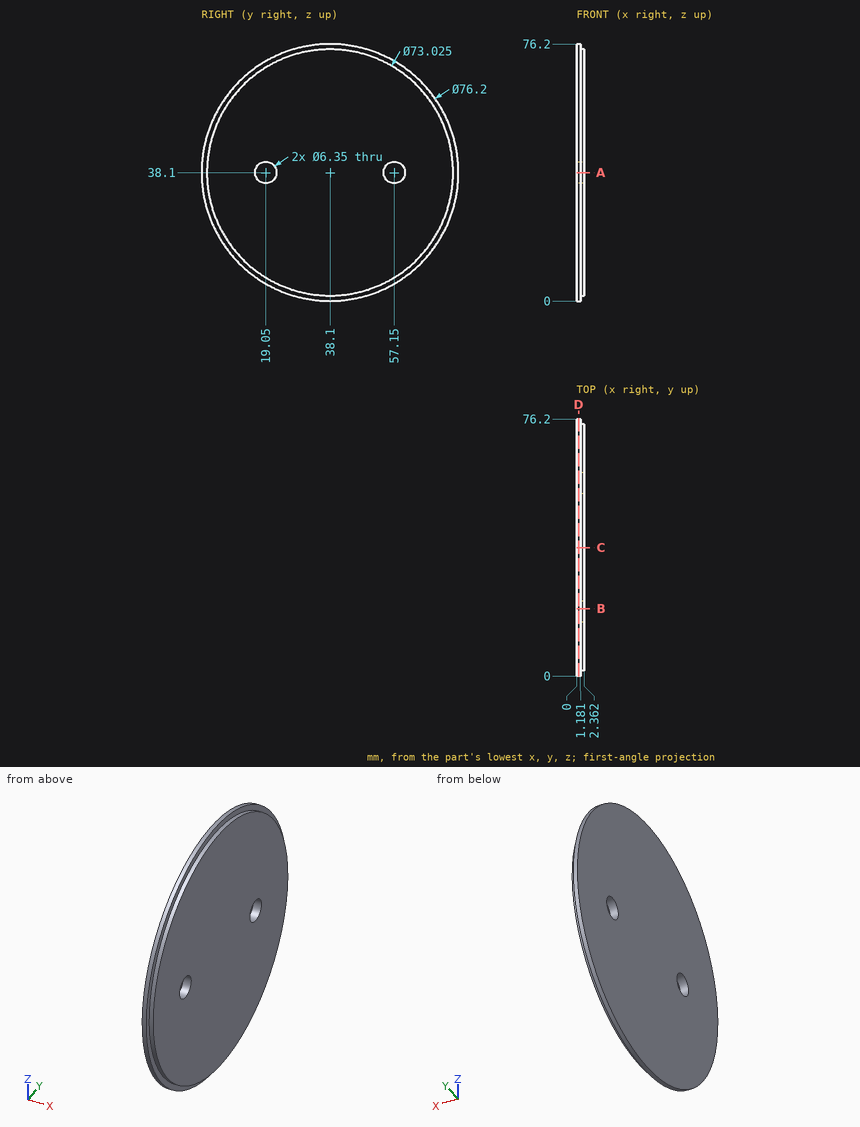
For this review, use the dimensioned drawing (mm, ordinates from the lowest corner) and the shaded views. Round coordinates to 2 decimals unless told otherwise and drop trailing zeros. Write each loop counter-clockwise with the first axis right and the second up, starting at its lowest first coordinate (ties: lowest second). Pieces come first, ordered by that corner, then holes. Notation, with made-up numbers: (84.25, 38.5) -> (121.25, 38.5) arc R35 cw to (121.25, 71.5) -> close; hole circle Ø4 at (-15.5, 87.25). An arc over 180 degrees is marked (long way). Use one line per item in the form item = value.
Q1. Consider section C-C (y = 38.1). State the section outline as (x, z) points.
Resolved:
outline = (0, 0) -> (1.18, 0) -> (1.18, 1.59) -> (2.36, 1.59) -> (2.36, 74.61) -> (1.18, 74.61) -> (1.18, 76.2) -> (0, 76.2) -> close
Q2. Consider section D-D (x = 0.6). State the section outline as (y, z) points (3 decimals), then the cut area to 3 significant figures.
Resolved:
outline = circle Ø76.2 at (38.1, 38.1); hole circle Ø6.35 at (19.05, 38.1); hole circle Ø6.35 at (57.15, 38.1)
area = 4,500 mm²
Q3. To check wall thickness, follow probe 1 along Y at (x, z) = (1.25, 38.1) (1 decimal); probe 2 along Y at (x, z) = (0.8, 38.1) (3 decimals); probe 3 along Z at (x, y) = (0.5, 18.5). State the ranges of each line that lie inside material, in increasing order. Write a range as from..to.
Resolved:
probe_1 = 1.6..15.9, 22.2..54, 60.3..74.6
probe_2 = 0..15.875, 22.225..53.975, 60.325..76.2
probe_3 = 5.43..34.97, 41.23..70.77
Q4. Consider section B-B (y = 20). State the section outline as (x, z) points, then the cut area to 3 significant figures.
Resolved:
outline = (0, 4.57) -> (1.18, 4.57) -> (1.18, 6.39) -> (2.36, 6.39) -> (2.36, 35.07) -> (0, 35.07) -> close; (0, 41.13) -> (2.36, 41.13) -> (2.36, 69.81) -> (1.18, 69.81) -> (1.18, 71.63) -> (0, 71.63) -> close
area = 140 mm²
Q5. Consider section A-A (z = 38.1). State the section outline as (x, y) points (1 decimal).
Resolved:
outline = (0, 0) -> (1.2, 0) -> (1.2, 1.6) -> (2.4, 1.6) -> (2.4, 15.9) -> (0, 15.9) -> close; (0, 22.2) -> (2.4, 22.2) -> (2.4, 54) -> (0, 54) -> close; (0, 60.3) -> (2.4, 60.3) -> (2.4, 74.6) -> (1.2, 74.6) -> (1.2, 76.2) -> (0, 76.2) -> close
